The listing builds one solid part. Answer for the finished solid, in the listing's coordinates (mm). A direction names the side the tool comes from. Give positions to 0.01 mm unless a question says otherwise; leave off trailing zeros. Order: outer loops, then holes, each group sorted by start corner. A loop starts at its lowest first (then second) coordinate and runs counter-clockwise, first axis right, second up. Notation, with made-up numbers: (-2.75, 76) - (23.25, 76) arc R25 cw to (23.25, 106) - close; hole circle Ø10 at (-1, -23). An arc over 180 degrees is marked (long way). Answer as a JSON object with one key per item and string values. Group by question number.
Q1. A cutting plane is placed at B-B, the plane z = -8.75. Give the vertices of the cut face in (x, y).
Q2. Given pin 1 (2 mm diameter, centred on x = -12.5, y = 19, fed in from +Z); pin 2 (4 mm diameter, centred on x = -10, y = 10.5, fed in from +Z); pin 3 (8 mm diameter, centred on x = -14.46, z = -6.75, fed in from -Y), each flat-ended and moving along its own axis, determine where each tip first touches the part or whether it passes through.
Q3. A cutting plane is placed at C-C, the plane y = 18.5. Give the vertices of the cut face in (x, z).
Q4. Consider line 1 (Y direction, x = -13, z = -9.75); line 2 (Y direction, x = -12.5, z = -1.5); line 3 (X direction, y = 22, z = -6.75). Determine where each line is inside the solid, lowest interval first.
Q5. A cutting plane is placed at D-D, the plane x = -20. Give the vertices of the cut face in (y, z).
Q6. The mould has two halves that part along Z. Classify faces 1 (the face through (-10.12, 0.99, -9.52)), 2 (the face through (-14, 2, -7)), 3 (the face through (-17.385, 25.134, -10.561)), 4 (the face through (-14, 33.5, -7)): released by +Z, released by -Z, zero draft, split by the parting line, or undercut.
Q7. A cutting plane is placed at A-A, the plane x = -12.75. Give the vertices of the cut face in (y, z), and give its area (3 significant figures).
Q8. For faces 5 (the face through (-14.4, 17, -1.8)), 6 (the face through (-21.835, 8.381, -8.388)), determine the directions among +Z, -Z, +X, -X, +Y, -Y from which every point of the face is accessible in a straight line to the end or side of a thin tool.
from build123d import *

# Parameters (mm, degrees)
SKETCH_1_R          = 7.55
EXTRUDE_1_DEPTH     = 17
SKETCH_2_R          = 5.15
CUT_EXTRUDE_1_DEPTH = 2
SKETCH_3_R          = 4.8
EXTRUDE_2_DEPTH     = 16.5


with BuildPart() as part:
    # 草图1 → 凸台-拉伸1 (new body)
    with BuildSketch(Plane(origin=(0, 0, 0), x_dir=(1, 0, 0), z_dir=(0, 1, 0))):
        with Locations(Location((-14.464315339, 6.751763544, 0), (0, 0, 270))):
            Circle(SKETCH_1_R)
    extrude(amount=EXTRUDE_1_DEPTH)

    # 草图2 → 切除-拉伸1 (cut)
    with BuildSketch(Plane.XZ):
        with Locations(Location((-14.464315339, -6.751763544, 0), (0, 0, 270))):
            Circle(SKETCH_2_R)
    extrude(amount=-CUT_EXTRUDE_1_DEPTH, mode=Mode.SUBTRACT)

    # 草图3 → 凸台-拉伸2 (add)
    with BuildSketch(Plane(origin=(0, 17, 0), x_dir=(1, 0, 0), z_dir=(0, 1, 0))):
        with Locations(Location((-14.464315339, 6.751763544, 0), (0, 0, 270))):
            Circle(SKETCH_3_R)
    extrude(amount=EXTRUDE_2_DEPTH)


solid = part.part
Reply:
{
 "1": {"outline": "(-21.75, 0) - (-19.21, 0) - (-19.21, 2) - (-9.72, 2) - (-9.72, 0) - (-7.18, 0) - (-7.18, 17) - (-10.1, 17) - (-10.1, 33.5) - (-18.83, 33.5) - (-18.83, 17) - (-21.75, 17) - close"},
 "2": {"pin 1": "stops at z = -2.05", "pin 2": "stops at z = 0.38", "pin 3": "stops at y = 2"},
 "3": {"outline": "circle Ø9.6 at (-14.46, -6.75)"},
 "4": {"line 1": "y = 2 to 33.5", "line 2": "y = 0 to 17", "line 3": "x = -19.26 to -9.66"},
 "5": {"outline": "(0, -11.89) - (17, -11.89) - (17, -1.62) - (0, -1.62) - close"},
 "6": {"face 1": "undercut", "face 2": "undercut", "face 3": "split by the parting line", "face 4": "zero draft"},
 "7": {"outline": "(0, -14.1) - (17, -14.1) - (17, -11.24) - (33.5, -11.24) - (33.5, -2.27) - (17, -2.27) - (17, 0.6) - (0, 0.6) - (0, -1.9) - (2, -1.9) - (2, -11.61) - (0, -11.61) - close", "area": "379 mm^2"},
 "8": {"face 5": "+Y", "face 6": "+Y, -Y"}
}
